Geometry: final body of the model. Coordinates: model frame, mm. Face numbers are marked on the shaded views. Give positions to 0.01 mm unless a question says otherwise; leave off trailing zeros. Write each loop counter-clockwise with the first axis right and the second up, starting at its lowest first coordinate (ties: lowest second). Pieces come first, ordered by that corner, then holes. Notation, with made-up numbers: M 7,-22.5 L 31,-22.5 A22 ccw 31,11.5 Z; hole C -4,15.5 d11. An arc over 180 degrees is marked long. One line per question, with ' | ' between items.
from build123d import *

# Parameters (mm, degrees)
EXTRUDE_1_DEPTH   = 2
HOLE_WIZARD_M81_D = 9
CHAMFER_1_SIZE    = 2


with BuildPart() as part:
    # Эскиз1 → Бобышка-Вытянуть1 (new body)
    with BuildSketch(Plane(origin=(0, 0, 0), x_dir=(1, 0, 0), z_dir=(0, 0, -1))):
        Polygon((0, 0), (0, 120), (120, 120), (120, 80), (40, 0), align=None)
    extrude(amount=EXTRUDE_1_DEPTH)

    # Отверстие с зазором M81 (through all)
    with Locations(Plane(origin=(0, 0, -2), x_dir=(1, 0, 0), z_dir=(0, 0, -1))):
        with Locations((60, 100), (20, 100), (20, 60), (20, 20), (100, 100), (60, 60)):
            Hole(HOLE_WIZARD_M81_D / 2)

    # Фаска1
    chamfer_1_edges = [part.edges().sort_by_distance(p)[0] for p in [
        (0, 0, -1),
        (0, -120, -1),
        (120, -120, -1),
    ]]
    chamfer(chamfer_1_edges, length=CHAMFER_1_SIZE)


solid = part.part
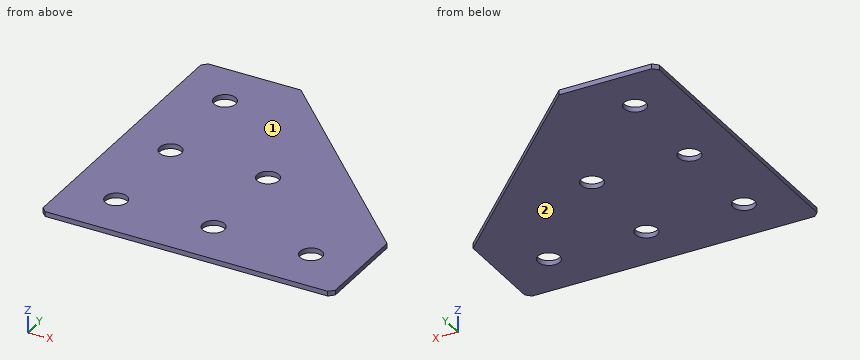
(1) Material intervals for L1, parallel to Y at x = 20, z = -0.6; L2, parallel to X at y = -100, z = -1.6; L3, parallel to Y at x = 60, z = -0.4, sorted ascending. Write a range as [from, to].
Working result:
L1: y = [-120, -104.5], [-95.5, -64.5], [-55.5, -24.5], [-15.5, 0] | L2: x = [0, 15.5], [24.5, 55.5], [64.5, 95.5], [104.5, 120] | L3: y = [-120, -104.5], [-95.5, -64.5], [-55.5, -20]
(2) Cut plane D-D, the plane y = -60. Return loops of the section in (x, z), then the cut area to 3 significant figures.
Working result:
outline: M 0,-2 L 15.5,-2 L 15.5,0 L 0,0 Z; M 24.5,-2 L 55.5,-2 L 55.5,0 L 24.5,0 Z; M 64.5,-2 L 100,-2 L 100,0 L 64.5,0 Z | area: 164 mm^2
(3) Draft query along Z for the marked faces 1 and 2. Return one class per face: released by +Z, released by -Z, zero draft, split by the parting line, or undercut.
Working result:
face 1: released by +Z | face 2: released by -Z
(4) First-contact query: P1, Ø8, axis at x = 100, y = -100, coming from the -Z side; P2, Ø10.5, axis at x = 60, y = -100, coming from the +Z side. Flat tips, straight axial feed; report the tip coordinate or a pass-through.
Working result:
P1: passes through | P2: stops at z = 0
(5) Cut plane A-A, the plane y = -100. Return loops of the section in (x, z), then the cut area to 3 significant figures.
Working result:
outline: M 0,-2 L 15.5,-2 L 15.5,0 L 0,0 Z; M 24.5,-2 L 55.5,-2 L 55.5,0 L 24.5,0 Z; M 64.5,-2 L 95.5,-2 L 95.5,0 L 64.5,0 Z; M 104.5,-2 L 120,-2 L 120,0 L 104.5,0 Z | area: 186 mm^2
(6) Cut plane B-B, the plane x = 20. Return loops of the section in (y, z), then the cut area to 3 significant figures.
Working result:
outline: M -120,-2 L -104.5,-2 L -104.5,0 L -120,0 Z; M -95.5,-2 L -64.5,-2 L -64.5,0 L -95.5,0 Z; M -55.5,-2 L -24.5,-2 L -24.5,0 L -55.5,0 Z; M -15.5,-2 L 0,-2 L 0,0 L -15.5,0 Z | area: 186 mm^2
(7) Cut plane C-C, the plane z = -1.3. Return loops of the section in (x, y).
Working result:
outline: M 0,-118 L 2,-120 L 118,-120 L 120,-118 L 120,-80 L 40,0 L 2,0 L 0,-2 Z; hole C 20,-100 d9; hole C 20,-60 d9; hole C 20,-20 d9; hole C 60,-100 d9; hole C 60,-60 d9; hole C 100,-100 d9
